Model file for the job. Use its own axes, mm. Face numbers are marked on the shaded views. Coordinates: 2 decimals unless noted, no trailing zeros. Write each loop counter-clockwise with the first axis right and the second up, starting at its lowest first coordinate (ties: lowest second). Pieces come first, ordered by that corner, then holes. Notation, with made-up numbers: M 55.5,25.25 L 112.5,25.25 A28 cw 112.5,60.25 Z; hole C 26.5,-9 d9. An arc over 180 degrees is marked long. Answer in a Markdown table with one row per item. Add a question column.
```python
from build123d import *

# Parameters (mm, degrees)
SKETCH1_W           = 40
SKETCH1_H           = 12
BOSS_EXTRUDE1_DEPTH = 3
SKETCH3_R           = 1.25
CUT_EXTRUDE2_DEPTH  = 22.09502311
CUT_EXTRUDE3_DEPTH  = 10
FILLET2_R           = 5
FILLET3_R           = 1
FILLET4_R           = 5
FILLET5_R           = 5
SKETCH6_W           = 35.954210482
SKETCH6_H           = 25.866097198
CUT_EXTRUDE4_DEPTH  = 10


with BuildPart() as part:
    # Sketch1 → Boss-Extrude1 (new body)
    with BuildSketch(Plane(origin=(0, 0, 0), x_dir=(1, 0, 0), z_dir=(0, 1, 0))):
        Rectangle(SKETCH1_W, SKETCH1_H)
    extrude(amount=BOSS_EXTRUDE1_DEPTH)

    # Sketch3 → Cut-Extrude2 (cut, through all)
    with BuildSketch(Plane(origin=(0, 3, 0), x_dir=(1, 0, 0), z_dir=(0, 1, 0))):
        with Locations(Location((-17.5, 3.5, 0), (0, 0, 270))):
            Circle(SKETCH3_R)
        with Locations(Location((-17.5, -3.5, 0), (0, 0, 270))):
            Circle(SKETCH3_R)
    extrude(amount=-CUT_EXTRUDE2_DEPTH, mode=Mode.SUBTRACT)

    # Sketch5 → Cut-Extrude3 (cut)
    with BuildSketch(Plane(origin=(0, 3, 0), x_dir=(1, 0, 0), z_dir=(0, 1, 0))):
        with BuildLine():
            Line((-13.458222524, 6), (20, 0))
            Line((20, 0), (20, -6))
            Line((20, -6), (17.030073052, -6))
            ThreePointArc((17.030073052, -6), (7.671541519, -2.617819669), (-2.144608615, -4.250134828))
            Line((-2.144608615, -4.250134828), (-6.569653649, -6))
            Line((-6.569653649, -6), (-13.458222524, -6))
            Line((-13.458222524, -6), (-13.458222524, -10.237178745))
            Line((-13.458222524, -10.237178745), (26.023482417, -9.726914384))
            Line((26.023482417, -9.726914384), (26.023482417, 8.477274399))
            Line((26.023482417, 8.477274399), (-13.458222524, 8.477274399))
            Line((-13.458222524, 8.477274399), (-13.458222524, 6))
        make_face()
    extrude(amount=-CUT_EXTRUDE3_DEPTH, mode=Mode.SUBTRACT)

    # Fillet2
    # the kernel refuses this fillet: 5 mm, written as the material it takes off along each edge
    with BuildSketch(Plane(origin=(-6.569653649, 5.381801612, 6), x_dir=(-1, 0, 0), z_dir=(0, -1, 0))) as fillet2_piece_1:
        with BuildLine():
            CenterArc((FILLET2_R * 0.190544128998, FILLET2_R), FILLET2_R, 248.423891744, 21.576108256)
            Line((-FILLET2_R * 0.17719268457, FILLET2_R * 0.0700700908417), (0, 0))
            Line((0, 0), (FILLET2_R * 0.190544128998, 0))
        make_face()
    extrude(amount=7.763603225, mode=Mode.SUBTRACT)
    with BuildSketch(Plane(origin=(-2.144608615, 3.259446384, 4.250134828), x_dir=(-0.9299299091583175, 0, 0.36773681356753396), z_dir=(0, -1, 0))) as fillet2_piece_2:
        with BuildLine():
            CenterArc((0.103778554, 5), FILLET2_R, 267.749266862, 2.250733138)
            ThreePointArc((-0.092584454, 0.003857331), (-0.046289955, 0.001983199), (0, 0))
            Line((0, 0), (0.103778554, 0))
        make_face()
    extrude(amount=3.518892769, mode=Mode.SUBTRACT)
    with BuildSketch(Plane(origin=(17.030073052, 6.64587884, 6), x_dir=(1, 0, 0), z_dir=(0, -1, 0))) as fillet2_piece_3:
        with BuildLine():
            CenterArc((1.458351536, -5), FILLET2_R, 90, 30.730822568)
            ThreePointArc((-1.096675494, -0.70211251), (-0.542524687, -0.360136055), (0, 0))
            Line((0, 0), (1.458351536, 0))
        make_face()
    extrude(amount=10.291757681, mode=Mode.SUBTRACT)

    # Fillet3
    fillet3_edges = [part.edges().sort_by_distance(p)[0] for p in [
        (20, 1.5, 6),
    ]]
    fillet(fillet3_edges, radius=FILLET3_R)

    # Fillet4
    fillet4_edges = [part.edges().sort_by_distance(p)[0] for p in [
        (20, 1.5, 0),
    ]]
    fillet(fillet4_edges, radius=FILLET4_R)

    # Fillet5
    fillet5_edges = [part.edges().sort_by_distance(p)[0] for p in [
        (-13.458222524, 1.5, -6),
    ]]
    fillet(fillet5_edges, radius=FILLET5_R)

    # Sketch6 → Cut-Extrude4 (cut)
    with BuildSketch(Plane(origin=(0, 3, 0), x_dir=(1, 0, 0), z_dir=(0, 1, 0))):
        with Locations((4.783435461, -3.359387953)):
            Rectangle(SKETCH6_W, SKETCH6_H)
    extrude(amount=-CUT_EXTRUDE4_DEPTH, mode=Mode.SUBTRACT)


solid = part.part
```
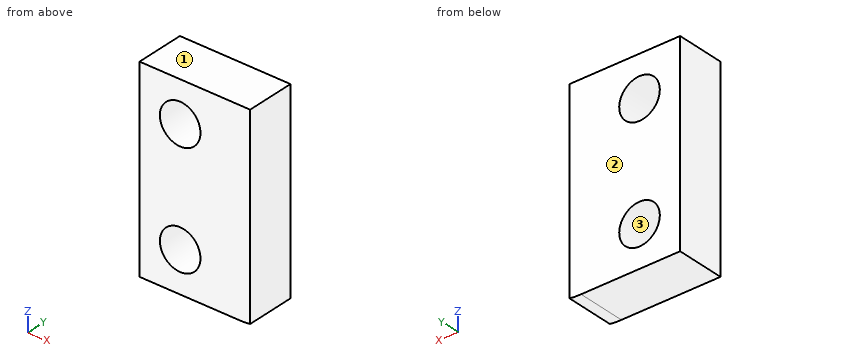
1) Slice it at D-D (x = -17.5). Give the cut face in (y, z), then the cut area to 3 significant figures.
2) Slice it at C-C (y = 2.05). Give the cut face in (x, z), then the cut area to 3 significant figures.
3) Slice it at B-B (z = 3.5). Give the cut face in (x, y), then the cut area to 3 significant figures.
4) Drill centre lines: probe 1 along X at (y, z) = (1.8, -3.5); probe 2 along Z at (x, y) = (-18.25, 0.3); probe 3 along Z at (x, y) = (-18, 1.9). Where is each one in solid material? Low to high.
5) Slice it at A-A (x = -18.25). Give the cut face in (y, z), then the cut area to 3 significant figures.
6) Two-plate mould, pull along Z, no slides. Class the marked faces 1, 2 and 3: released by +Z, released by -Z, zero draft, split by the parting line, or undercut.
Ans:
| question | item | result |
|---|---|---|
| 1 | outline | M 0,-6 L 3,-6 L 3,-4.75 L 0,-4.75 Z; M 0,-2.25 L 3,-2.25 L 3,2.25 L 0,2.25 Z; M 0,4.75 L 3,4.75 L 3,6 L 0,6 Z |
| 1 | area | 21.0 mm2 |
| 2 | outline | M -20,-6 L -13.9,-6 A5 ccw -13.19,-5.95 L -13.19,6 L -20,6 Z; hole C -17.5,-3.5 d2.5; hole C -17.5,3.5 d2.5 |
| 2 | area | 71.8 mm2 |
| 3 | outline | M -20,0 L -18.75,0 L -18.75,3 L -20,3 Z; M -16.25,0 L -13.19,0 L -13.19,3 L -16.25,3 Z |
| 3 | area | 12.9 mm2 |
| 4 | probe 1 | x = -20 to -18.75, -16.25 to -13.19 |
| 4 | probe 2 | z = -6 to -4.5, -2.5 to 2.5, 4.5 to 6 |
| 4 | probe 3 | z = -6 to -4.65, -2.35 to 2.35, 4.65 to 6 |
| 5 | outline | M 0,-6 L 3,-6 L 3,-4.5 L 0,-4.5 Z; M 0,-2.5 L 3,-2.5 L 3,2.5 L 0,2.5 Z; M 0,4.5 L 3,4.5 L 3,6 L 0,6 Z |
| 5 | area | 24.0 mm2 |
| 6 | face 1 | released by +Z |
| 6 | face 2 | zero draft |
| 6 | face 3 | undercut |
